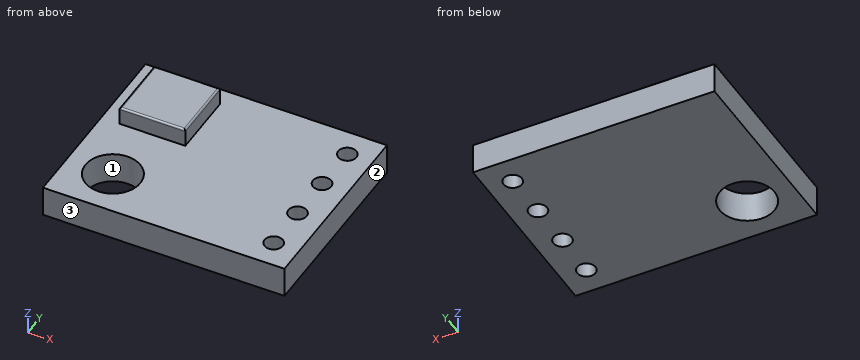
from build123d import *

# Parameters (mm, degrees)
F0_W     = 13.2
F0_H     = 10.62
F1_DEPTH = 1.7
F2_R     = 0.5
F2_R_2   = 1.5
F3_DEPTH = 1.701
F4_W     = 3.6
F4_H     = 3.6
F5_DEPTH = 1
F6_R     = 0.1


with BuildPart() as f1:
    # F0 (on Top) → F1 (new body)
    with BuildSketch(Plane.XY):
        Rectangle(F0_W, F0_H)
    extrude(amount=F1_DEPTH)

    # F2 (on face) → F3 (cut, through all)
    with BuildSketch(Plane.XY.offset(1.7)):
        with Locations((5.222315, 3.81)):
            Circle(F2_R)
        with Locations((5.182661, 1.27)):
            Circle(F2_R)
        with Locations((5.182661, -1.27)):
            Circle(F2_R)
        with Locations((5.222315, -3.81)):
            Circle(F2_R)
        with Locations((-4.1, -2.81)):
            Circle(F2_R_2)
    extrude(amount=-F3_DEPTH, mode=Mode.SUBTRACT)

    # F4 (on face) → F5 (join)
    with BuildSketch(Plane.XY.offset(1.7)):
        with Locations((-3.8, 2.51)):
            Rectangle(F4_W, F4_H)
    extrude(amount=F5_DEPTH)

    # F6
    f6_edges = [f1.edges().sort_by_distance(p)[0] for p in [
        (-3.8, 0.71, 2.7),
        (-2, 2.51, 2.7),
        (-5.6, 2.51, 2.7),
        (-3.8, 4.31, 2.7),
    ]]
    fillet(f6_edges, radius=F6_R)


solid = f1.part
Geometry: final body of the model. Coordinates: model frame, mm. Face numbers are marked on the shaded views. Round coordinates to 2 decimals unless told otherwise and drop trailing zeros. Write each loop counter-clockwise with the first axis right and the second up, starting at its lowest first coordinate (ties: lowest second). Pieces come first, ordered by that corner, then holes. Notation, with made-up numbers: M 11,-23.5 L 29,-23.5 A12 ccw 29,-9.5 Z; hole C 77.5,46.5 d4. An arc over 180 degrees is marked long. Write item = value, one per line.
Item 1: Section query C-C on y = 2.75. Return loops of the section in (x, z), then the cut area to 3 significant figures.
Findings:
outline = M -6.6,0 L 6.6,0 L 6.6,1.7 L -2,1.7 L -2,2.6 A0.1 ccw -2.1,2.7 L -5.5,2.7 A0.1 ccw -5.6,2.6 L -5.6,1.7 L -6.6,1.7 Z
area = 26.0 mm^2
Item 2: Pin query (flat end, axial travel): P1, Ø2.5, axis at x = -4.1, y = -2.81, coming from the +Z side. Return the tip coordinate at first contact, or that it passes through.
Findings:
P1 = through
Item 3: Section query A-A on y = -2.81. Return loops of the section in (x, z), then the cut area to 3 significant figures.
Findings:
outline = M -6.6,0 L -5.6,0 L -5.6,1.7 L -6.6,1.7 Z; M -2.6,0 L 6.6,0 L 6.6,1.7 L -2.6,1.7 Z
area = 17.3 mm^2
Item 4: Section query D-D on y = -1. Return loops of the section in (x, z), then the cut area to 3 significant figures.
Findings:
outline = M -6.6,0 L 4.76,0 L 4.76,1.7 L -6.6,1.7 Z; M 5.6,0 L 6.6,0 L 6.6,1.7 L 5.6,1.7 Z
area = 21.0 mm^2
Item 5: Pull-direction query (X, two-part tool) for the marked faces 1, 2 and 3; classes: pulls with the +X half, pulls with the -X half, needs draft (parallel to the pull), parting line crosses it, or undercut.
Findings:
face_1 = undercut
face_2 = pulls with the +X half
face_3 = needs draft
Item 6: Section query B-B on z = 1. Return loops of the section in (x, y).
Findings:
outline = M -6.6,-5.31 L 6.6,-5.31 L 6.6,5.31 L -6.6,5.31 Z; hole C -4.1,-2.81 d3; hole C 5.18,-1.27 d1; hole C 5.18,1.27 d1; hole C 5.22,-3.81 d1; hole C 5.22,3.81 d1
Item 7: Material intervals for line 1 along X through (y, z) = (1.25, 1.6); line 2 along Z through (x, y) = (3.5, 0.75); line 3 along Y through (x, z) = (-2.75, 0.9), sorted ascending. Write a range as [from, to].
Findings:
line_1 = [-6.6, 4.68], [5.68, 6.6]
line_2 = [0, 1.7]
line_3 = [-5.31, -3.46], [-2.16, 5.31]
